Design review of the part built by this model. Coordinates are the model's own, in mm. A direction names the side the tool comes from. Give positions to 0.01 mm unless a question says otherwise; leave off trailing zeros. Loops run counter-clockwise (first coordinate to the right, second up) from the corner with the lowest first, then second, coordinate; pieces in that order, holes last. Notation, with made-up numbers: (-17, 31) - (-8, 31) arc R11 cw to (-8, 49) - close; hole circle Ø9 at (28.5, 86). An arc over 180 degrees is marked (long way). Write each question's results on one line, items separated by ' | '.
Autodesk Inventor part; units mm, degrees
ref_plane "YZ Plane" through (0, 0, 0) normal (1, 0, 0) x (0, 1, 0)
ref_plane "XZ Plane" through (0, 0, 0) normal (0, 1, 0) x (-1, 0, 0)
ref_plane "XY Plane" through (0, 0, 0) normal (0, 0, 1) x (1, 0, 0)
ref_plane "РабПлоскость1" through (0, 0, 0) normal (0, 0, 1) x (1, 0, 0)
sketch "Эскиз1" plane through (0, 0, 0) normal (0, 0, 1) x (1, 0, 0)
  line L0 (15.9535, 22.685) -> (15.9535, 17.285)
  line L1 (15.9535, 17.285) -> (5.5535, 17.285)
  line L2 (5.5535, 17.285) -> (5.5535, 22.685)
  line L3 (5.5535, 22.685) -> (15.9535, 22.685)
  line L4 (15.9535, -17.315) -> (15.9535, -22.715)
  line L5 (15.9535, -22.715) -> (5.5535, -22.715)
  line L6 (5.5535, -22.715) -> (5.5535, -17.315)
  line L7 (5.5535, -17.315) -> (15.9535, -17.315)
  arc A0 (-2.3465, 28.685) -> (-4.3465, 26.685) centre (-2.3465, 26.685) ccw
  line L8 (-4.3465, 12.1) -> (-4.3465, 26.685)
  arc A1 (-5.6809, 10.2141) -> (-4.3465, 12.1) centre (-6.3465, 12.1) ccw
  line L9 (-11.5122, 8.156) -> (-5.6809, 10.2141)
  arc A2 (-11.5122, 8.156) -> (-12.8465, 6.27) centre (-10.8465, 6.27) ccw
  line L10 (-12.8465, -1.915) -> (-12.8465, 6.27)
  arc A3 (-12.8465, -1.915) -> (-10.8465, -3.915) centre (-10.8465, -1.915) ccw
  line L11 (-4.6465, -3.915) -> (-10.8465, -3.915)
  arc A4 (-2.6465, -5.915) -> (-4.6465, -3.915) centre (-4.6465, -5.915) ccw
  line L12 (-2.6465, -26.715) -> (-2.6465, -5.915)
  arc A5 (-2.6465, -26.715) -> (-0.6465, -28.715) centre (-0.6465, -26.715) ccw
  line L13 (23.8535, -28.715) -> (-0.6465, -28.715)
  arc A6 (23.8535, -28.715) -> (25.8535, -26.715) centre (23.8535, -26.715) ccw
  line L14 (25.8535, 26.685) -> (25.8535, -26.715)
  arc A7 (25.8535, 26.685) -> (23.8535, 28.685) centre (23.8535, 26.685) ccw
  line L15 (-2.3465, 28.685) -> (23.8535, 28.685)
  circle A8 centre (18.0535, 25.685) radius 0.8
  circle A9 centre (21.6535, 25.685) radius 0.8
  circle A10 centre (21.6535, -25.715) radius 0.8
  circle A11 centre (18.0535, -25.715) radius 0.8
  circle A12 centre (0.3535, -18.515) radius 0.8
  circle A13 centre (0.3535, -14.915) radius 0.8
  circle A14 centre (-1.3465, 16.885) radius 0.8
  circle A15 centre (-1.3465, 20.485) radius 0.8
  circle A16 centre (-0.1465, 25.685) radius 0.8
  circle A17 centre (3.4535, 25.685) radius 0.8
  circle A18 centre (-0.1465, -25.715) radius 0.8
  circle A19 centre (3.4535, -25.715) radius 0.8
  line L16 (-4.3465, 12.1) -> (-2.6465, -5.915)
  circle A20 centre (51.6035, 35.685) radius 3
  circle A21 centre (51.6035, 35.685) radius 6
  line L17 (11.6035, -28.715) -> (11.6035, 28.685) construction
  line L18 (56.9244, 32.9123) -> (25.8535, -26.715)
  line L19 (50.1799, 41.5137) -> (-2.3465, 28.685)
  point P0 (0, 0)
  point P1 (-2.6818, -5.5409)
  dimension "d11" = 6
  dimension "d12" = 12
  dimension "d13" = 7
  dimension "d14" = 40
extrude "Выдавливание1" add sketch "Эскиз1" along normal blind 2.5 contours L0 L1 L2 L3 | L4 L5 L6 L7 | L15 A7 L14 A6 L13 A5 L12 A4 L16 L8 A0
ref_plane "РабПлоскость4" through (0, 0, 12.5) normal (0, 0, 1) x (1, 0, 0)
sketch "Эскиз7" plane through (0, 0, 12.5) normal (0, 0, 1) x (1, 0, 0)
  circle A0 centre (11.6035, 42.685) radius 3
  circle A1 centre (11.6035, 42.685) radius 7
  line L0 (18.3597, 40.8537) -> (15.6035, 30.685)
  line L1 (15.6035, 30.685) -> (15.6035, 10.685)
  line L2 (15.6035, 10.685) -> (7.6035, 10.685)
  line L3 (7.6035, 10.685) -> (7.6035, 30.685)
  line L4 (7.6035, 30.685) -> (4.8473, 40.8537)
  line L5 (-0.6465, -28.715) -> (23.8535, -28.715)
  line L6 (11.6035, -28.715) -> (11.6035, 28.685) construction
  line L7 (23.8535, 28.685) -> (-2.3465, 28.685)
  point P0 (0, 0)
  point P1 (11.6035, 10.685)
  dimension "d46" = 6
  dimension "d47" = 14
  dimension "d48" = 32
  dimension "d49" = 4
  dimension "d50" = 18
  dimension "d51" = 20
  dimension "d52" = 20
extrude "Выдавливание5" add sketch "Эскиз7" along normal blind 2.5
ref_plane "РабПлоскость5" through (11.6035, 10.685, 12.5) normal (1, 0, 0) x (0, 0, -1)
sketch "Эскиз8" plane through (11.6035, 10.685, 12.5) normal (1, 0, 0) x (0, 0, -1)
  line L0 (0, 20) -> (0, 30.1687)
  line L1 (10, 18) -> (10, 16)
  line L2 (0, 20) -> (10, 18)
  line L3 (-2.5, 20) -> (-2.5, 0)
  line L4 (-2.5, 0) -> (10, -23)
  line L5 (10, -37.4) -> (10, 16)
  line L6 (0, 0) -> (0, 20)
  line L7 (0, 0) -> (-2.5, 0)
  line L8 (0, 20) -> (0, 0)
  line L9 (0, 0) -> (10, -18.4)
  line L10 (10, -16.6) -> (10, -37.4)
  line L11 (0, 17.4505) -> (10, 15.4505)
  line L12 (10, 16) -> (10, 1.415)
  line L13 (12.5, 18) -> (10, 18)
  line L14 (10, 18) -> (0, 25.5)
  point P0 (12.5, -10.685)
  dimension "d55" = 23
  dimension "d56" = 2.5
  dimension "d61" = 5.5
extrude "Выдавливание6" add sketch "Эскиз8" along normal mid plane 2.5 contours L0 L14 L2 | L11 L5 L9 L6
extrude "Выдавливание7" add sketch "Эскиз8" along normal mid plane 8 contours L2 L1 L5 L11 L6 | L9 L5 L4 L7
properties part number "Fastener"
Item 1: Clearance check with flat-ended pins moving along their axes: P1, Ø1.2, axis at y = -15, z = 1.5, coming from the -X side; P2, Ø8, axis at y = -2.5, z = 8, coming from the -X side; P3, Ø1.5, axis at x = 19.5, z = 3, coming from the +Y side (3 decimals). State where each tip first meets the part, or that it passes through.
Output values:
P1: stops at x = -2.65 | P2: stops at x = 7.6 | P3: stops at y = 28.685
Item 2: We need section D-D on y = 2. Give the boundary of the cut face in (x, z), then the cut area to 3 significant figures.
Output values:
outline: (-3.39, 0) - (25.85, 0) - (25.85, 2.5) - (12.85, 2.5) - (12.85, 7.78) - (15.6, 7.78) - (15.6, 10.28) - (7.6, 10.28) - (7.6, 7.78) - (10.35, 7.78) - (10.35, 2.5) - (-3.39, 2.5) - close | area: 106 mm²
Item 3: Tool access review of faces 4 (the face through (12, 38, 12.5)), 5 (the face through (10.354, 14, 8)), 6 (the face through (15.604, 14, 13)), 7 (the face through (12.854, 14, 8)): name each direction out of +Z, -Z, +X, -X, +Y, -Y from which nothing blocks a thin tool from reaching the whole face with its end or side.
Output values:
face 4: -Z, +Y | face 5: -X | face 6: +Z, +X, -Y | face 7: +X
Item 4: Wall thickness on probe 1 along Y at (x, z) = (0.5, 1) (3 decimals); probe 2 along Z at (x, y) = (24.5, -19); probe 3 along X at (y, z) = (16.5, 12): over which ranges is each line inside the solid? List them lowest first.
Output values:
probe 1: y = -28.715 to -26.186, -25.244 to -19.301, -17.729 to -15.701, -14.129 to 25.214, 26.156 to 28.685 | probe 2: z = 0 to 2.5 | probe 3: x = 10.35 to 12.85
Item 5: We need section C-C on z = 5.75. Give the boundary of the cut face in (x, y) (1 decimal).
Output values:
outline: (7.6, -6.3) - (15.6, -6.3) - (15.6, -1.7) - (12.9, -1.7) - (12.9, 26.8) - (15.6, 26.8) - (15.6, 29.3) - (12.9, 29.3) - (12.9, 31.1) - (10.4, 31.1) - (10.4, 29.3) - (7.6, 29.3) - (7.6, 26.8) - (10.4, 26.8) - (10.4, -1.7) - (7.6, -1.7) - close
Item 6: We need section A-A on y = 44. Give the boundary of the cut face in (x, z).
Output values:
outline: (4.73, 12.5) - (8.91, 12.5) - (8.91, 15) - (4.73, 15) - close; (14.3, 12.5) - (18.48, 12.5) - (18.48, 15) - (14.3, 15) - close
Item 7: We need section B-B on y = 13.5. Give the boundary of the cut face in (x, z).
Output values:
outline: (-4.35, 0) - (25.85, 0) - (25.85, 2.5) - (12.85, 2.5) - (12.85, 12.5) - (15.6, 12.5) - (15.6, 15) - (7.6, 15) - (7.6, 12.5) - (10.35, 12.5) - (10.35, 2.5) - (-4.35, 2.5) - close
Item 8: Draft analysis for pull direction X (two halves, no side actions). For faces 1 (the face through (14.21, 1.61, 7.57)), 2 (the face through (3.3, -26.5, 1.2)), 3 (the face through (25.252, 28.115, 1.232)), state which applies: +X half, -X half, draft (parallel to the pull), parting line (faces both ways), or undercut.
Output values:
face 1: draft | face 2: undercut | face 3: +X half
